Geometry: final body of the model. Coordinates: model frame, mm. Face numbers are marked on the shaded views. A direction names the side the tool comes from. Give positions to 0.01 mm unless a question says otherwise; leave off trailing zeros. Order: outer loops, then holes, each group sorted by start corner. A loop starts at its lowest first (then second) coordinate and runs counter-clockwise, first axis right, second up. Notation, with made-up numbers: (74, 88) - (88, 88) arc R20 cw to (88, 120) - close; hole circle Ø4 at (74, 1.5). An arc over 180 degrees is marked (long way). Use one line per item in the form item = value.
from build123d import *

# Parameters (mm, degrees)
F0_W     = 47.5073454976
F0_H     = 4
F0_W_2   = 8
F0_H_2   = 30
F1_DEPTH = 15
F3_R     = 10.286668946
F4_DEPTH = 10
F6_DEPTH = 10


with BuildPart() as f1:
    # F0 (on Front) → F1 (new body)
    with BuildSketch(Plane.XZ):
        Polygon((37.5, -17.5), (37.5, -2.5), (29.5, -2.5), (29.5, -13.5), (29.5, -17.5), align=None)
        with Locations((5.7463272512, -15.5)):
            Rectangle(F0_W, F0_H)
        Polygon((37.5, 2.5), (-37.5, 2.5), (-37.5, -2.5), (-29.5, -2.5), (29.5, -2.5), (37.5, -2.5), align=None)
        with Locations((-33.5, -17.5)):
            Rectangle(F0_W_2, F0_H_2)
    extrude(amount=F1_DEPTH)

    # F2: F1 across plane


with BuildPart() as f1_1:
    add(f1.part)
    add(f1.part.mirror(Plane.XZ))

    # F3 (on face) → F4 (cut)
    with BuildSketch(Plane(origin=(0, 0, -17.5), x_dir=(1, 0, 0), z_dir=(0, 0, -1))):
        Circle(F3_R)
    extrude(amount=-F4_DEPTH, mode=Mode.SUBTRACT)

    # F5 (on face) → F6 (cut)
    with BuildSketch(Plane(origin=(-37.5, 0, 0), x_dir=(0, -1, 0), z_dir=(-1, 0, 0))):
        with BuildLine():
            ThreePointArc((8.5, -16), (6.0104076401, -9.9895923599), (0, -7.5))
            ThreePointArc((0, -7.5), (-6.0104076401, -22.0104076401), (8.5, -16))
        make_face()
    extrude(amount=-F6_DEPTH, mode=Mode.SUBTRACT)


solid = f1_1.part
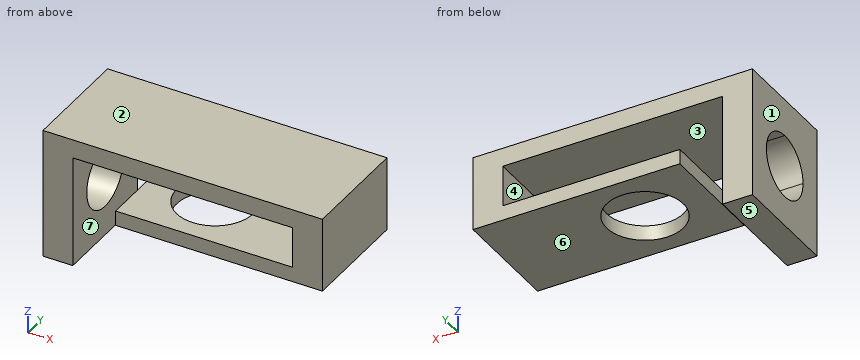
(1) Cut plane A-A on x = -13. Output: boundary loops of the cut face in (y, z), plus the area to 3 significant figures.
Computed values:
outline = (-15, -17.5) - (15, -17.5) - (15, -13.5) - (-15, -13.5) - close; (-15, -2.5) - (15, -2.5) - (15, 2.5) - (-15, 2.5) - close
area = 270 mm²
(2) Pull-direction query (X, two-part tool) for the marked faces 1, 2 and 3; classes: released by +X, released by -X, zero draft, split by the parting line, or undercut.
Computed values:
face_1 = released by -X
face_2 = zero draft
face_3 = undercut
(3) Cut plane D-D on y = 0.75. Output: boundary loops of the cut face in (x, z).
Computed values:
outline = (-37.5, -32.5) - (-29.5, -32.5) - (-29.5, -24.47) - (-37.5, -24.47) - close; (-37.5, -7.53) - (-29.5, -7.53) - (-29.5, -2.5) - (29.5, -2.5) - (29.5, -13.5) - (10.26, -13.5) - (10.26, -17.5) - (37.5, -17.5) - (37.5, 2.5) - (-37.5, 2.5) - close; (-18.01, -17.5) - (-10.26, -17.5) - (-10.26, -13.5) - (-18.01, -13.5) - close
(4) Cut plane C-C on x = 0. Output: boundary loops of the cut face in (y, z).
Computed values:
outline = (-15, -17.5) - (-10.29, -17.5) - (-10.29, -13.5) - (-15, -13.5) - close; (-15, -2.5) - (15, -2.5) - (15, 2.5) - (-15, 2.5) - close; (10.29, -17.5) - (15, -17.5) - (15, -13.5) - (10.29, -13.5) - close
(5) Cut plane B-B on z = -4. Output: boundary loops of the cut face in (x, y), plus the area to 3 significant figures.
Computed values:
outline = (-37.5, -15) - (-29.5, -15) - (-29.5, 15) - (-37.5, 15) - close; (29.5, -15) - (37.5, -15) - (37.5, 15) - (29.5, 15) - close
area = 480 mm²
(6) Contact query for a flat-ended pin moving along its axis: pin 1 Ø4.5 at (y, z) = (2, -16) entering from -X. Output: stop coordinate, or through.
Computed values:
pin_1 = -18.01
(7) Ray query, line 1 along X through (y, z) = (7.75, -7); line 2 along Z through (x, y) = (-13, -3.25); line 3 along X through (y, z) = (0, -14.3). Return the intervals inside material, ascending.
Computed values:
line_1 = -37.5 to -29.5, 29.5 to 37.5
line_2 = -17.5 to -13.5, -2.5 to 2.5
line_3 = -18.01 to -10.29, 10.29 to 37.5
(8) Reachability of the marked faces 4, 5, 6 and 7 from +Z, -Z, +X, -X, +Y, -Y: full face, straight path, thin tool, end or side. Return the list, or none.
Computed values:
face_4 = +Y, -Y
face_5 = -Z, +X, -X, +Y, -Y
face_6 = -Z, +X, +Y, -Y
face_7 = -Z, +Y, -Y
